Read the model definition and answer for the solid it produces. Units are mm, in the model's axes. Face numbers are marked on the shaded views. A direction names the side the tool comes from. Give positions to 0.01 mm unless a question says otherwise; leave off trailing zeros. Order: outer loops, then holes, each group sorted by start corner. A loop starts at its lowest first (then second) coordinate and runs counter-clockwise, first axis right, second up. Notation, with made-up numbers: (25.25, 61) - (60.25, 61) arc R12 ccw to (60.25, 81) - close; hole circle Ø8 at (48, 70). An arc over 180 degrees is marked (long way). One line per item, written item: value. Start each with the question number.
```python
from build123d import *

# Parameters (mm, degrees)
SKETCH_2_R          = 2.5
CUT_EXTRUDE_1_DEPTH = 62.846584384


with BuildPart() as part:
    # 草图1 → 旋转2 (revolve)
    with BuildSketch(Plane.XY):
        Polygon((0, 30), (0, 0), (45, 0), (45, 5), (25, 5), (25, 6), (15, 6), (15, 10), (5, 10), (5, 30), align=None)
    revolve(axis=Axis((45, 0, 0), (-1, 0, 0)))

    # 草图2 → 切除-拉伸1 (cut, through all)
    with BuildSketch(Plane.ZY):
        with Locations(Location((0, 22.5, 0), (0, 0, 270))):
            Circle(SKETCH_2_R)
        with Locations(Location((19.485571585, 11.25, 0), (0, 0, 270))):
            Circle(SKETCH_2_R)
        with Locations(Location((19.485571585, -11.25, 0), (0, 0, 270))):
            Circle(SKETCH_2_R)
        with Locations(Location((0, -22.5, 0), (0, 0, 270))):
            Circle(SKETCH_2_R)
        with Locations(Location((-19.485571585, -11.25, 0), (0, 0, 270))):
            Circle(SKETCH_2_R)
        with Locations(Location((-19.485571585, 11.25, 0), (0, 0, 270))):
            Circle(SKETCH_2_R)
    extrude(amount=-CUT_EXTRUDE_1_DEPTH, mode=Mode.SUBTRACT)


solid = part.part
```
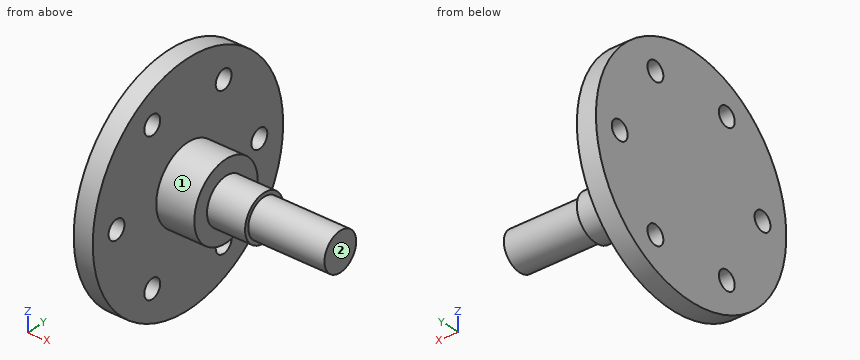
1) Section B-B on y = -23.5 is taken. Write down the section's boundary in (x, z).
2) Section C-C on y = 0 is taken. Write down the section's boundary in (x, z).
3) Section D-D on x = 27 is taken. Write down the section's boundary in (y, z).
4) Each of these flat-tipped pins is pushed along its axis until it touches: pin 1 (10 mm diameter, centred on x = 5, y = -17.5, fed in from +Z); pin 2 (12 mm diameter, centred on x = 5, z = 9, fed in from +Y); pin 3 (4 mm diameter, centred on y = 2, z = -22.5, fed in from -X); pin 4 (1.5 mm diameter, centred on x = 32, y = -3.5, fed in from +Z). Where does it stop, or does it pass through?
5) Find the intervals of material crossed by probe 1 along Z at (x, y) = (1.45, -11.25); probe 2 along Z at (x, y) = (3, -11); probe 3 along X at (y, z) = (-0.5, 6.5), in increasing order. Write a range as from..to.
6) Section A-A on y = 11.25 is taken. Write down the section's boundary in (x, z).
7) For the marked faces 1 and 2, determine the directions among +Z, -Z, +X, -X, +Y, -Y from which every point of the face is accessible in a straight line to the end or side of a thin tool.
Solved:
1. outline: (0, -18.65) - (5, -18.65) - (5, -2.29) - (0, -2.29) - close; (0, 2.29) - (5, 2.29) - (5, 18.65) - (0, 18.65) - close
2. outline: (0, -30) - (5, -30) - (5, -10) - (15, -10) - (15, -6) - (25, -6) - (25, -5) - (45, -5) - (45, 5) - (25, 5) - (25, 6) - (15, 6) - (15, 10) - (5, 10) - (5, 30) - (0, 30) - close
3. outline: circle Ø10 at (0, 0)
4. pin 1: stops at z = 27.27
4. pin 2: stops at y = 29.85
4. pin 3: stops at x = 0
4. pin 4: stops at z = 4.18
5. probe 1: z = -27.81..-21.99, -16.99..16.99, 21.99..27.81
5. probe 2: z = -27.91..-21.97, -17..17, 21.97..27.91
5. probe 3: x = 0..15
6. outline: (0, -27.81) - (5, -27.81) - (5, -21.99) - (0, -21.99) - close; (0, -16.99) - (5, -16.99) - (5, 16.99) - (0, 16.99) - close; (0, 21.99) - (5, 21.99) - (5, 27.81) - (0, 27.81) - close
7. face 1: +X
7. face 2: +Z, -Z, +X, +Y, -Y
